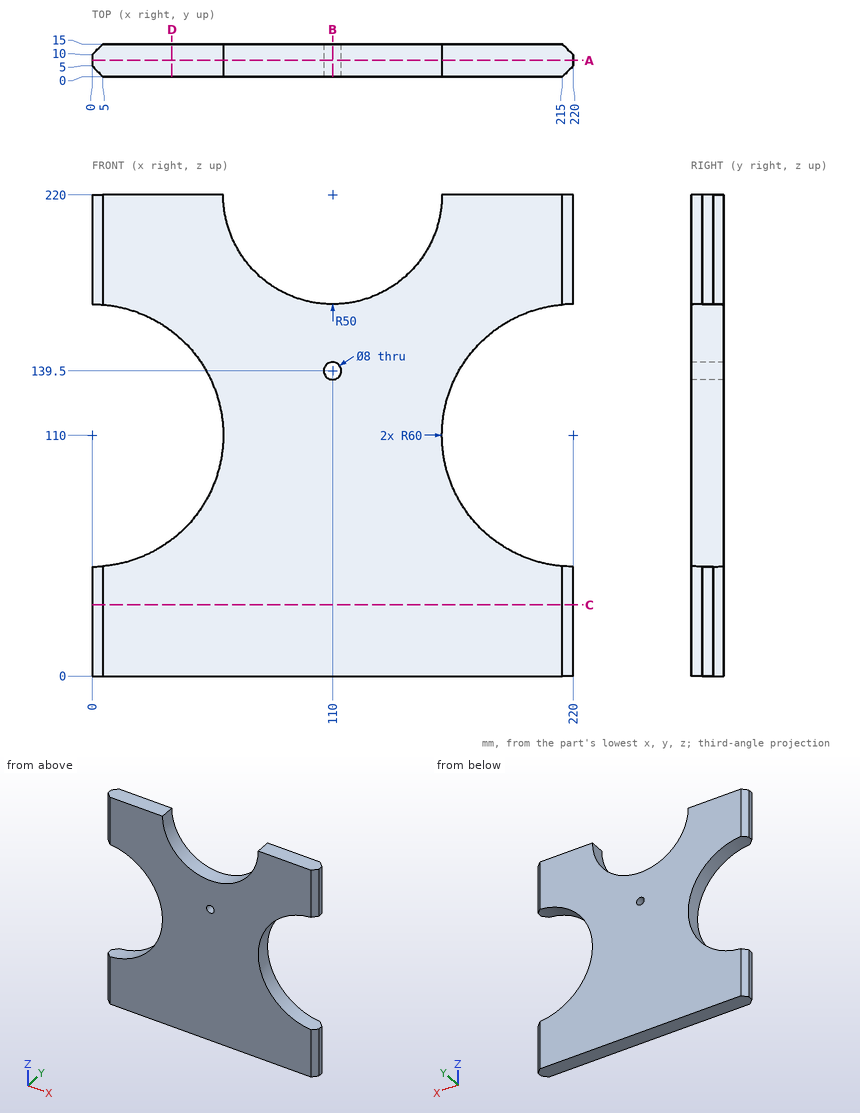
Study the drawing (mm; zero at the part's minimum x, y, z) and answer. Coordinates: 2 decimals unless noted, no trailing zeros. Loops run counter-clockwise (first coordinate to the right, second up) from the corner with the lowest first, then second, coordinate; pieces in that order, holes last. Notation, with made-up numbers: M 64,-32 L 113,-32 A12 ccw 113,-17 Z; hole C 79,-40 d8. An arc over 180 degrees is marked long. Answer as a JSON object with one key per item and string values. Group by question number.
Item 1: Each of these flat-tipped pins is pushed along its axis until it touches: P1, Ø6, axis at x = 147.5, y = 8, coming from the +Z side; P2, Ø4, axis at y = 5.5, z = 69, coming from the +X side; P3, Ø8, axis at y = 2, z = 123, coming from the +X side. Where does it stop, or does it pass through?
Item 2: Section B-B (x = 110) is taken. Write down the section's boundary in (y, z).
Item 3: Section A-A (y = 7.5) is taken. Write down the section's boundary in (x, z).
Item 4: Section C-C (z = 32.5) is taken. Write down the section's boundary in (x, y), and give its area (3 significant figures).
Item 5: Section D-D (x = 36.5) is taken. Write down the section's boundary in (y, z), and give its area (3 significant figures).
Item 6: Consider L1, parallel to Z at x = 110, y = 9; L2, parallel to X at y = 4.25, z = 139.5; L3, parallel to Z at x = 32, y = 1. Determine where each line is inside the solid, lowest interval first.
Solved:
{
 "1": {"P1": "stops at z = 190.68", "P2": "stops at x = 178.16", "P3": "stops at x = 162.46"},
 "2": {"outline": "M 0,0 L 15,0 L 15,135.5 L 0,135.5 Z; M 0,143.5 L 15,143.5 L 15,170 L 0,170 Z"},
 "3": {"outline": "M 0,0 L 220,0 L 220,50 A60 cw 220,170 L 220,220 L 160,220 A50 cw 60,220 L 0,220 L 0,170 A60 cw 0,50 Z; hole C 110,139.5 d8"},
 "4": {"outline": "M 0,5 L 5,0 L 215,0 L 220,5 L 220,10 L 215,15 L 5,15 L 0,10 Z", "area": "3,250 mm2"},
 "5": {"outline": "M 0,0 L 15,0 L 15,62.38 L 0,62.38 Z; M 0,157.62 L 15,157.62 L 15,220 L 0,220 Z", "area": "1,870 mm2"},
 "6": {"L1": "z = 0 to 135.5, 143.5 to 170", "L2": "x = 52.25 to 106, 114 to 167.75", "L3": "z = 0 to 59.25, 160.75 to 220"}
}
